Work out the finished part from the listing and answer in its coordinate system (mm). Face numbers are marked on the shaded views. A direction names the side the tool comes from. Give positions to 0.01 mm unless a question says otherwise; leave off trailing zeros. Write each loop counter-clockwise with the first axis right and the second up, starting at its lowest first coordinate (ties: lowest second). Pieces come first, ordered by that corner, then holes. Notation, with made-up numbers: (63, -30) -> (68, -30) arc R13 cw to (68, -26) -> close; hole circle Ø4 at (-5, 53). An arc over 180 degrees is marked (long way). Use a Markdown table: item, result. Add a question column.
Q1. Section A-A, the plane x = 52.5 is taken. Give the vertices of the cut face in (y, z).
Q2. For a pull along Y with two mould halves and no side action, classify the marked faces 3, 4, 5 and 6 as pulls with the +Y half, pulls with the -Y half, needs draft (parallel to the pull), parting line crosses it, or undercut.
Q3. For the marked faces 1 and 2, determine the directions among +Z, -Z, +X, -X, +Y, -Y from which every point of the face is accessible in a straight line to the end or side of a thin tool.
Q4. Each of these flat-tipped pins is pushed along its axis until it touches: pin 1 Ø2 at (y, z) = (-10, 21.5) entering from -X; pin 2 Ø1.5 at (x, z) = (20.5, 18.5) entering from -Y. Where does it stop, or does it pass through?
Q5. Consider line 1 (Y direction, x = 12.7, z = 20); line 2 (X direction, y = -13.5, z = 9); line 3 (X direction, y = -15.75, z = 4). Determine where each line is inside the solid, lowest interval first.
Q6. Section C-C, the plane y = -18 is taken. Give the vertices of the cut face in (x, z), plus the area to 3 significant figures.
Q7. Section B-B, the plane z = 21 is taken. Give the vertices of the cut face in (x, y).
Q8. Section D-D, the plane z = 2 is taken. Give the vertices of the cut face in (x, y), plus the area to 3 significant figures.
from build123d import *

# Parameters (mm, degrees)
F1_DEPTH = 25.4
F3_DEPTH = 12.701
F5_DEPTH = 38.101
F7_DEPTH = 25.4


with BuildPart() as f1:
    # F0 (on Front) → F1 (new body)
    with BuildSketch(Plane.XZ):
        Polygon((0, 38.1), (0, 0), (76.2, 0), (76.2, 12.7), (25.4, 12.7), (25.4, 38.1), align=None)
    extrude(amount=F1_DEPTH)

    # F2 (on face) → F3 (cut, through all)
    with BuildSketch(Plane.XY.offset(12.7)):
        with BuildLine():
            Line((76.2, 0), (63.5, 0))
            ThreePointArc((63.5, 0), (75.756906611, -12.7), (63.5, -25.4))
            Line((63.5, -25.4), (76.2, -25.4))
            Line((76.2, -25.4), (76.2, 0))
        make_face()
        with BuildLine():
            ThreePointArc((69.85, -12.7), (67.9901280605, -8.2098719395), (63.5, -6.35))
            Line((63.5, -6.35), (63.5, -19.05))
            ThreePointArc((63.5, -19.05), (67.9901280605, -17.1901280605), (69.85, -12.7))
        make_face()
        with BuildLine():
            Line((63.5, -19.05), (63.5, -6.35))
            ThreePointArc((63.5, -6.35), (57.15, -12.7), (63.5, -19.05))
        make_face()
        with BuildLine():
            ThreePointArc((63.5, -19.05), (57.15, -12.7), (63.5, -6.35))
            Line((63.5, -6.35), (38.1, -6.35))
            ThreePointArc((38.1, -6.35), (42.5901280605, -8.2098719395), (44.45, -12.7))
            ThreePointArc((44.45, -12.7), (42.5901280605, -17.1901280605), (38.1, -19.05))
            Line((38.1, -19.05), (63.5, -19.05))
        make_face()
        with BuildLine():
            Line((38.1, -19.05), (38.1, -6.35))
            ThreePointArc((38.1, -6.35), (31.75, -12.7), (38.1, -19.05))
        make_face()
        with BuildLine():
            ThreePointArc((44.45, -12.7), (42.5901280605, -8.2098719395), (38.1, -6.35))
            Line((38.1, -6.35), (38.1, -19.05))
            ThreePointArc((38.1, -19.05), (42.5901280605, -17.1901280605), (44.45, -12.7))
        make_face()
    extrude(amount=-F3_DEPTH, mode=Mode.SUBTRACT)

    # F4 (on face) → F5 (cut, through all)
    with BuildSketch(Plane.XY.offset(38.1)):
        with BuildLine():
            ThreePointArc((0, -12.7), (3.7197438789, -3.7197438789), (12.7, 0))
            Line((12.7, 0), (0, 0))
            Line((0, 0), (0, -12.7))
        make_face()
        with BuildLine():
            Line((0, -25.4), (12.7, -25.4))
            ThreePointArc((12.7, -25.4), (3.7197438789, -21.6802561211), (0, -12.7))
            Line((0, -12.7), (0, -25.4))
        make_face()
        with BuildLine():
            ThreePointArc((6.35, -12.7), (12.7, -19.05), (19.05, -12.7))
            Line((19.05, -12.7), (6.35, -12.7))
        make_face()
        with BuildLine():
            Line((6.35, -12.7), (19.05, -12.7))
            ThreePointArc((19.05, -12.7), (12.7, -6.35), (6.35, -12.7))
        make_face()
    extrude(amount=-F5_DEPTH, mode=Mode.SUBTRACT)

    # F6 (on face) → F7 (cut)
    with BuildSketch(Plane.XY.offset(38.1)):
        with BuildLine():
            Line((25.4, -25.4), (25.4, -12.7))
            ThreePointArc((25.4, -12.7), (21.6802561211, -21.6802561211), (12.7, -25.4))
            Line((12.7, -25.4), (25.4, -25.4))
        make_face()
        with BuildLine():
            ThreePointArc((12.7, 0), (21.6802561211, -3.7197438789), (25.4, -12.7))
            Line((25.4, -12.7), (25.4, 0))
            Line((25.4, 0), (12.7, 0))
        make_face()
    extrude(amount=-F7_DEPTH, mode=Mode.SUBTRACT)


solid = f1.part
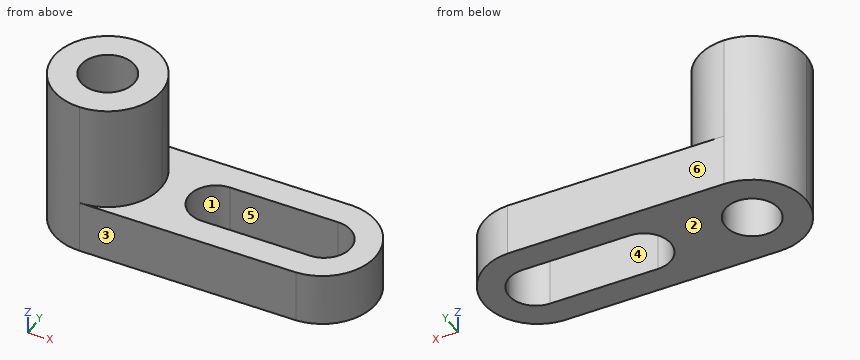
Result set:
| question | item | result |
|---|---|---|
| 1 | outline | (-25.4, 0) -> (-19.05, 0) -> (-19.05, 12.7) -> (-25.4, 12.7) -> close; (-6.35, 0) -> (0, 0) -> (0, 12.7) -> (-6.35, 12.7) -> close |
| 2 | face 3 | pulls with the -Y half |
| 2 | face 4 | undercut |
| 2 | face 5 | undercut |
| 2 | face 6 | pulls with the +Y half |
| 3 | face 1 | +Z, -Z |
| 3 | face 2 | -Z, +X, -X, +Y, -Y |
| 4 | pin 1 | stops at x = 0.11 |
| 4 | pin 2 | stops at y = -23.26 |
| 5 | line 1 | y = -25.4 to -19.05, -6.35 to 0 |
| 5 | line 2 | x = 0.03 to 6.4, 19 to 31.8, 69.8 to 75.73 |
| 5 | line 3 | x = 0.37 to 7.13, 18.27 to 32.53, 69.07 to 75.39 |
| 6 | outline | (1.16, 0) -> (9.2, 0) -> (9.2, 38.1) -> (1.16, 38.1) -> close; (16.2, 0) -> (34.6, 0) -> (34.6, 12.7) -> (24.24, 12.7) -> (24.24, 38.1) -> (16.2, 38.1) -> close; (67, 0) -> (74.6, 0) -> (74.6, 12.7) -> (67, 12.7) -> close |
| 6 | area | 841 mm2 |
| 7 | outline | circle Ø25.4 at (12.7, -12.7); hole circle Ø12.7 at (12.7, -12.7) |
| 8 | outline | (12.7, -25.4) -> (63.5, -25.4) arc R12.71 ccw to (63.5, 0) -> (12.7, 0) arc R12.7 ccw to start; hole circle Ø12.7 at (12.7, -12.7); hole (38.1, -19.05) -> (63.5, -19.05) arc R6.35 ccw to (63.5, -6.35) -> (38.1, -6.35) arc R6.35 ccw to start |
| 8 | area | 1,210 mm2 |
